Geometry: final body of the model. Coordinates: model frame, mm. Give positions to 0.01 mm unless a question says otherwise; leave off trailing zeros. Write each loop counter-clockwise with the first axis right and the second up, starting at its lowest first coordinate (ties: lowest second). Pieces come first, ordered by that corner, then holes. Notation, with made-up numbers: M 35.25,58.25 L 93.25,58.25 A8 ccw 93.25,73.25 Z; hole C 64.25,-16.5 d9. An arc over 180 degrees is marked long. Use a Markdown table: item, result. Add a question column.
(1) Pin query (flat end, axial travel): pin 1 Ø2.5 at (x, y) = (137, 20) entering from -Z; pin 2 Ø5.5 at (x, y) = (122.73, 31.89) entering from +Z; pin 3 Ø6 at (x, y) = (435.5, 26.5) entering from -Z. Return the tip coordinate at first contact, or that it passes through.
(2) Cut plane A-A (z = 20.75). Output: boundary loops of the cut face in (x, y) (3 decimals), plus the area to 3 significant figures.
(3) Material intervals for L1, parallel to Y at x = 121, z = 18.25; L2, parallel to Z at x = 422, y = 33, sorted ascending.
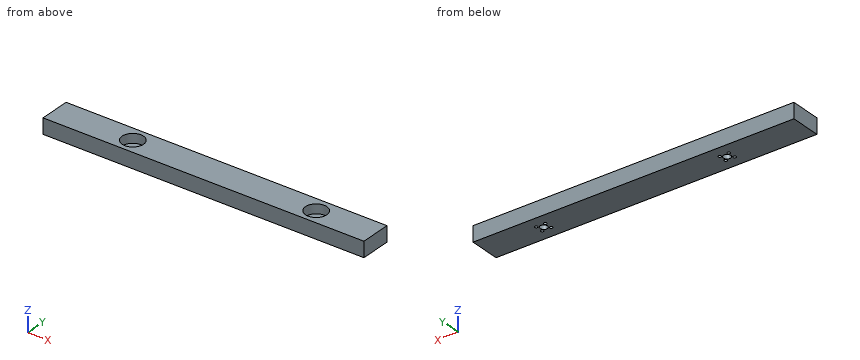
```python
from build123d import *

# Parameters (mm, degrees)
SKETCH1_W           = 533.4
SKETCH1_H           = 50.8
BOSS_EXTRUDE1_DEPTH = 25.4
CUT_EXTRUDE1_START  = -10.16
SKETCH3_R           = 17.78
CUT_EXTRUDE1_DEPTH  = 127
SKETCH4_R           = 6.0198
SKETCH4_R_2         = 2.4638
CUT_EXTRUDE2_DEPTH  = 7.62


with BuildPart() as part:
    # Sketch1 → Boss-Extrude1 (new body)
    with BuildSketch(Plane.XY):
        with Locations((266.7, 25.4)):
            Rectangle(SKETCH1_W, SKETCH1_H)
    extrude(amount=BOSS_EXTRUDE1_DEPTH)

    # Sketch3 → Cut-Extrude1 (cut)
    with BuildSketch(Plane(origin=(0, 0, 0), x_dir=(-1, 0, 0), z_dir=(0, 0, -1)).offset(CUT_EXTRUDE1_START)):
        with Locations((-130.175, 25.290721308)):
            Circle(SKETCH3_R)
        with Locations((-434.975, 25.290721308)):
            Circle(SKETCH3_R)
    extrude(amount=-CUT_EXTRUDE1_DEPTH, mode=Mode.SUBTRACT)

    # Sketch4 → Cut-Extrude2 (cut)
    with BuildSketch(Plane(origin=(0, 0, 0), x_dir=(-1, 0, 0), z_dir=(0, 0, -1))):
        with Locations((-130.175, 25.4)):
            Circle(SKETCH4_R)
        with Locations((-122.728486169, 18.909255319)):
            Circle(SKETCH4_R_2)
        with Locations((-122.728486169, 31.890744681)):
            Circle(SKETCH4_R_2)
        with Locations((-137.621513831, 18.909255319)):
            Circle(SKETCH4_R_2)
        with Locations((-137.621513831, 31.890744681)):
            Circle(SKETCH4_R_2)
        with Locations((-434.975, 25.4)):
            Circle(SKETCH4_R)
        with Locations((-427.528486169, 18.909255319)):
            Circle(SKETCH4_R_2)
        with Locations((-427.528486169, 31.890744681)):
            Circle(SKETCH4_R_2)
        with Locations((-442.421513831, 18.909255319)):
            Circle(SKETCH4_R_2)
        with Locations((-442.421513831, 31.890744681)):
            Circle(SKETCH4_R_2)
    extrude(amount=-CUT_EXTRUDE2_DEPTH, mode=Mode.SUBTRACT)


solid = part.part
```
Answer list:
| question | item | result |
|---|---|---|
| 1 | pin 1 | z = 0 |
| 1 | pin 2 | z = 10.16 |
| 1 | pin 3 | z = 7.62 |
| 2 | outline | M 0,0 L 533.4,0 L 533.4,50.8 L 0,50.8 Z; hole C 130.175,25.291 d35.56; hole C 434.975,25.291 d35.56 |
| 2 | area | 25,100 mm² |
| 3 | L1 | 0 to 10.06, 40.52 to 50.8 |
| 3 | L2 | 0 to 10.16 |
